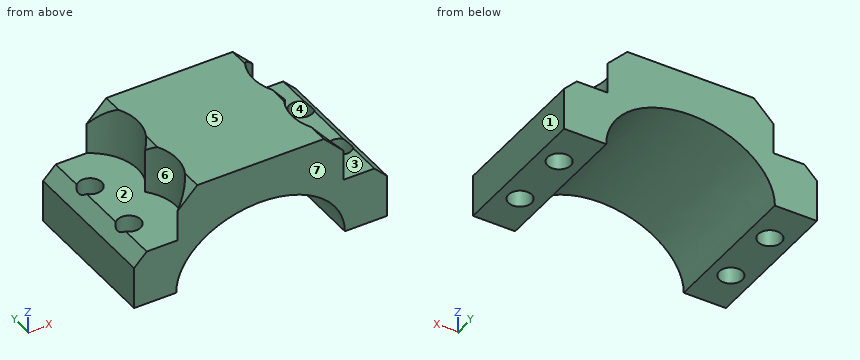
from build123d import *

# Parameters (mm, degrees)
PAD025_DEPTH        = 35
HOLE025_D           = 5.5
HOLE025_DEPTH       = 25
HOLE025_CBORE_D     = 22.6
HOLE025_CBORE_DEPTH = 12
HOLE025_TIPS_R      = 2.75
POCKET001_DEPTH     = 48


with BuildPart() as part:
    # Sketch054 → Pad025 (new body)
    with BuildSketch(Plane.XZ):
        with BuildLine():
            Line((50, -1e-05), (60, 0))
            Line((60, 0), (60, 25))
            Line((60, 25), (0, 25))
            Line((0, 25), (0, 0))
            Line((0, 0), (10, 5e-06))
            add(Edge.make_bspline(
                [(30, 15), (10.000006, 15), (10, 5e-06)],
                knots=[4.712389, 4.712389, 4.712389, 6.283185, 6.283185, 6.283185], degree=2, weights=[1, 0.707107, 1]))
            add(Edge.make_bspline(
                [(50, -1e-05), (50.000013, 15), (30, 15)],
                knots=[3.141592, 3.141592, 3.141592, 4.712389, 4.712389, 4.712389], degree=2, weights=[1, 0.707107, 1]))
        make_face()
    extrude(amount=PAD025_DEPTH)

    # Hole025
    with Locations(Plane.XY.offset(25)):
        with Locations((55, -25), (55, -10), (5, -25), (5, -10)):
            CounterBoreHole(HOLE025_D / 2, HOLE025_CBORE_D / 2, HOLE025_CBORE_DEPTH, depth=HOLE025_DEPTH)

    # Hole025 tips → Hole025 tip 1 section 0
    with BuildSketch(Plane.XY, mode=Mode.PRIVATE) as hole025_tip_1_s0:
        with Locations((55, -25)):
            Circle(HOLE025_TIPS_R)
    loft([hole025_tip_1_s0.sketch, Vertex(55, -25, -1.652367)], mode=Mode.SUBTRACT)

    # Hole025 tips → Hole025 tip 2 section 0
    with BuildSketch(Plane.XY, mode=Mode.PRIVATE) as hole025_tip_2_s0:
        with Locations((55, -10)):
            Circle(HOLE025_TIPS_R)
    loft([hole025_tip_2_s0.sketch, Vertex(55, -10, -1.652367)], mode=Mode.SUBTRACT)

    # Hole025 tips → Hole025 tip 3 section 0
    with BuildSketch(Plane.XY, mode=Mode.PRIVATE) as hole025_tip_3_s0:
        with Locations((5, -25)):
            Circle(HOLE025_TIPS_R)
    loft([hole025_tip_3_s0.sketch, Vertex(5, -25, -1.652367)], mode=Mode.SUBTRACT)

    # Hole025 tips → Hole025 tip 4 section 0
    with BuildSketch(Plane.XY, mode=Mode.PRIVATE) as hole025_tip_4_s0:
        with Locations((5, -10)):
            Circle(HOLE025_TIPS_R)
    loft([hole025_tip_4_s0.sketch, Vertex(5, -10, -1.652367)], mode=Mode.SUBTRACT)

    # Sketch056 → Pocket001 (cut)
    with BuildSketch(Plane.XZ):
        Polygon((60, 10), (40, 30), (60, 30), align=None)
        Polygon((20, 30), (0, 10), (0, 30), align=None)
    extrude(amount=POCKET001_DEPTH, mode=Mode.SUBTRACT)


with BuildPart() as part_1:
    # Body057 placement: moved
    add(part.part.moved(Location((55, 65, 40))))


solid = part_1.part
Input: part model. Units: mm. Frame: model coordinates. Face numbers are marked on the shaded views. A direction names the side the tool comes from. Coordinates: 2 decimals unless noted, no trailing zeros. Order: outer loops, then holes, each group sorted by start corner. A loop starts at its lowest first (then second) coordinate and runs counter-clockwise, first axis right, second up. Notation, with made-up numbers: M -13,62.5 L 9,62.5 A22 ccw 9,99.5 Z; hole C 47,76.5 d9. An arc over 180 degrees is marked long. Write item = value, one per line. Start each with the question number.
(1) First-contact query: P1, Ø1.5, axis at x = 100.5, y = 48, coming from the -Z side; P2, Ø4, axis at x = 84.5, y = 50, coming from the -Z side; P3, Ø7, axis at x = 110, y = 40, coming from the -Z side; P4, Ø7, axis at x = 60, y = 55, coming from the +Z side. Flat tips, straight axial feed; report the tip coordinate or a pass-through.
(2) Section C-C on z = 56.5. Output: boundary loops of the cut face in (x, y), and give its area (3 significant figures).
(3) Section A-A on x = 60. Output: boundary loops of the cut face in (y, z), and give its area (3 significant figures).
(4) Section B-B on z = 42. Give the number of separate pieces and of enclosed holes in the cut face, and give its area (3 significant figures).
(5) Reachability of the marked faces 1, 2 and 3 from +Z, -Z, +X, -X, +Y, -Y: full face, straight path, thin tool, end or side. Return the list, or none.
(6) Line query: line 1 along Y through (x, z) = (60, 50); line 2 along X through (y, z) = (40, 50); line 3 along X through (y, z) = (55, 45.5). Output: solid intervals per line, ascending. Write a range as [from, to].
(7) Pull-direction query (Y, two-part tool) for the marked faces 4, 5, 6 and 7; classes: released by +Y, released by -Y, zero draft, split by the parting line, or undercut.
Result set:
q1.P1 = 48.74
q1.P2 = 54.88
q1.P3 = 40
q1.P4 = 53
q2.outline = M 65.26,30 L 104.74,30 A11.3 cw 101.55,47.5 A11.3 cw 104.74,65 L 65.26,65 A11.3 cw 68.45,47.5 A11.3 cw Z
q2.area = 1,060 mm²
q3.outline = M 30,40 L 37.25,40 L 37.25,53 L 30,53 Z; M 42.75,40 L 52.25,40 L 52.25,53 L 42.75,53 Z; M 57.75,40 L 65,40 L 65,53 L 57.75,53 Z
q3.area = 312 mm²
q4.separate_pieces = 2
q4.enclosed_holes = 4
q4.area = 617 mm²
q5.face_1 = +Z, -Z, +X, +Y, -Y
q5.face_2 = +Z, -X
q5.face_3 = +Z, +X
q6.line_1 = [30, 37.25], [42.75, 52.25], [57.75, 65]
q6.line_2 = [55, 57.25], [62.75, 70.09], [99.91, 107.25], [112.75, 115]
q6.line_3 = [55, 57.25], [62.75, 66.39], [103.61, 107.25], [112.75, 115]
q7.face_4 = undercut
q7.face_5 = zero draft
q7.face_6 = undercut
q7.face_7 = released by -Y
